Could you check a few things on this drawing? It's one solid part, dimensions in mm from its lowest x, y, z. Round coordinates to 2 decimals unless told otherwise and drop trailing zeros. Loops run counter-clockwise (first coordinate to the right, second up) from the corner with the lowest first, then second, coordinate; pieces in that order, holes last. Notation, with made-up numbers: M -23,-39 L 5,-39 A21 cw 5,-31 Z; hole C 70,43.5 d10. An arc over 180 degrees is marked long. Answer as a JSON object with one key per item and string values.
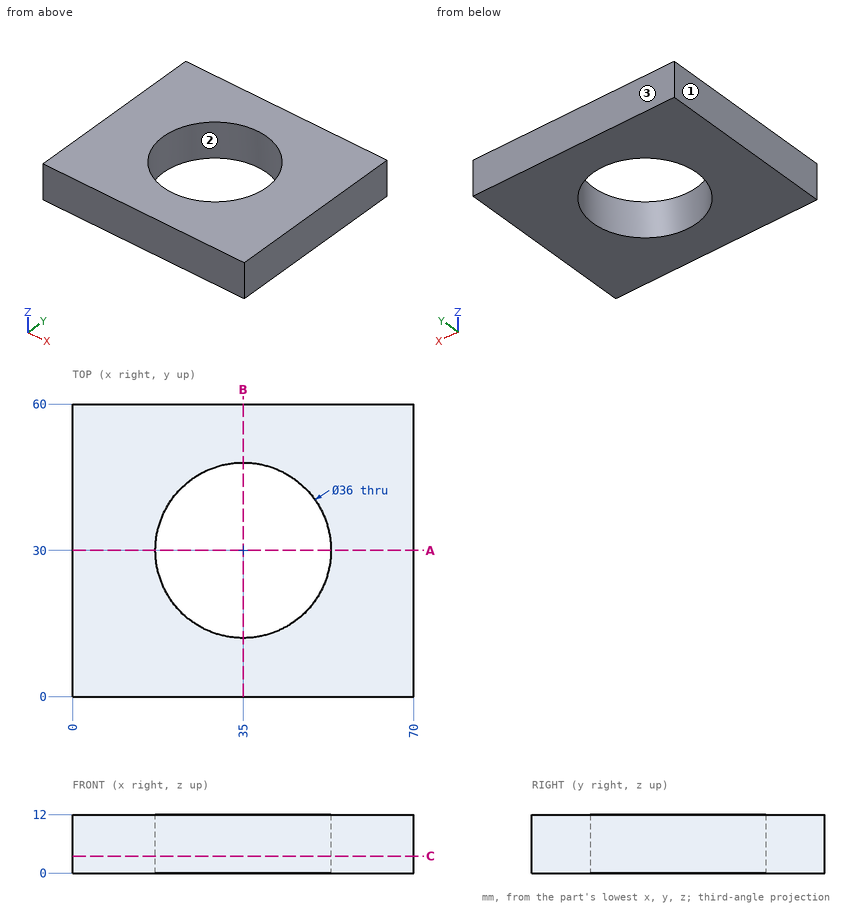
Item 1: I want a section at B-B, the plane x = 35. Please give me the cut outline in (y, z).
Resolved:
{"outline": "M 0,0 L 12,0 L 12,12 L 0,12 Z; M 48,0 L 60,0 L 60,12 L 48,12 Z"}
Item 2: I want a section at A-A, the plane y = 30. Please give me the cut outline in (x, z), then the cut area to 3 significant figures.
Resolved:
{"outline": "M 0,0 L 17,0 L 17,12 L 0,12 Z; M 53,0 L 70,0 L 70,12 L 53,12 Z", "area": "408 mm²"}
Item 3: Please list where these lines run through material, in increasing order: probe 1 along Y at (x, z) = (35, 6.5); probe 2 along X at (y, z) = (25.5, 8.75); probe 3 along X at (y, z) = (21.5, 7). Write a range as from..to.
Resolved:
{"probe 1": "0..12, 48..60", "probe 2": "0..17.57, 52.43..70", "probe 3": "0..19.13, 50.87..70"}
Item 4: If we mould it in two halves opening along Y, with no side actions, what happens to the marked faces 1, 2 and 3? For each: pulls with the +Y half, pulls with the -Y half, needs draft (parallel to the pull), parting line crosses it, or undercut.
Resolved:
{"face 1": "needs draft", "face 2": "undercut", "face 3": "pulls with the +Y half"}
Item 5: I want a section at C-C, the plane z = 3.5. Please give me the cut outline in (x, y).
Resolved:
{"outline": "M 0,0 L 70,0 L 70,60 L 0,60 Z; hole C 35,30 d36"}
